Answer from the drawing. Dimensions are ordinates in mm from the lowest x, y and z of the part. A direction names the side the tool comes from. Coordinates: 2 decimals unless noted, no trailing zeros. Order: outer loops, then holes, each group sorted by start corner. A loop starts at its lowest first (then second) coordinate and runs counter-clockwise, first axis right, second up. Notation, with made-up numbers: M -34.5,6 L -30.5,6 A19 cw -30.5,34 Z; hole C -6,-26.75 d8. An arc over 180 degrees is marked long. One line per question, with ' | ' between items. Start each with the question number.
1) Find section A-A, the plane y = 5.61. Write down the section's boundary in (x, z).
2) Given P1, Ø7, axis at x = 19.31, y = 18.29, coming from the -Z side; P2, Ø3.5, axis at x = 6.63, y = 18.29, coming from the -Z side; P3, Ø6, axis at x = 25.5, z = 4, coming from the +Y side, each flat-ended and moving along its own axis, determine where each tip first touches the part or whether it passes through.
3) Find section B-B, the plane x = 31.99. Write down the section's boundary in (y, z), plus the area to 3 significant figures.
4) Consider probe 1 along Y at (x, z) = (31.99, 12.75); probe 2 along Z at (x, y) = (34, 21.75); probe 3 along Y at (x, z) = (25, 1.5). Determine where each line is inside the solid, lowest interval first.
5) Find section D-D, the plane x = 10. Write down the section's boundary in (y, z).
6) Find section C-C, the plane z = 8.25. Write down the section's boundary in (x, y).
7) A tool of negligible diameter and unlimited length cuts with its end or side. For the marked faces 1 and 2, from which of +Z, -Z, +X, -X, +Y, -Y can it reach the whole face along a straight path? Write none if from no direction.
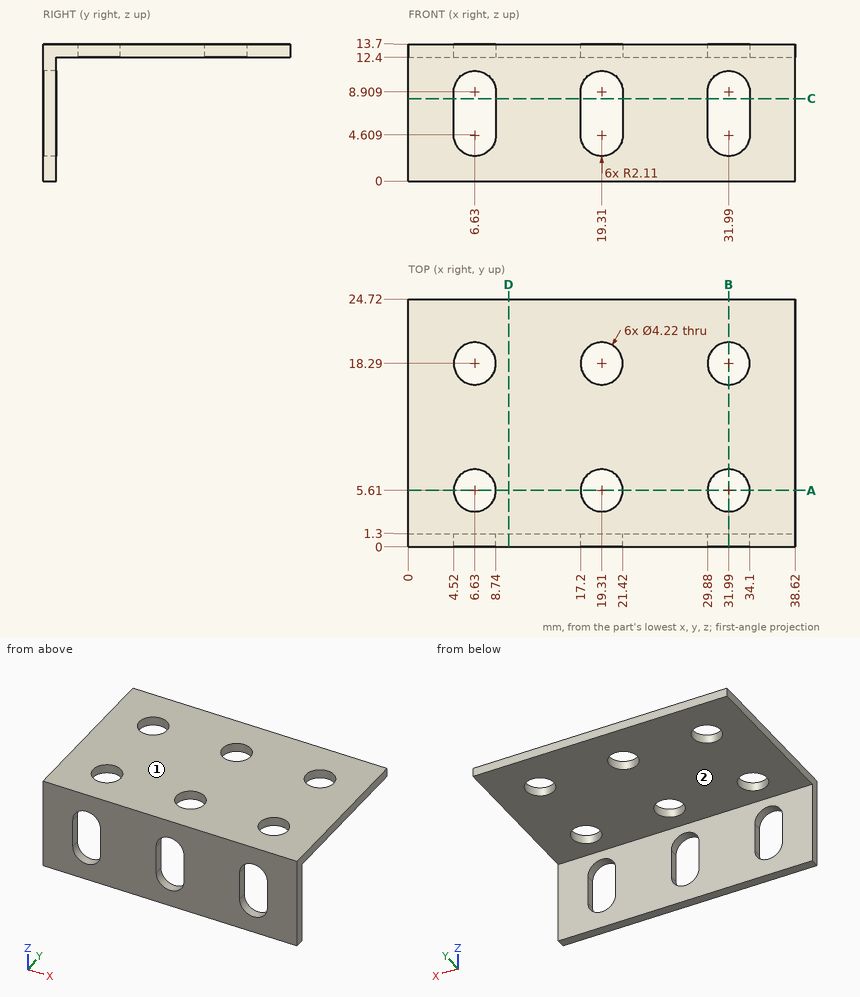
Report:
1) outline: M 0,12.4 L 4.52,12.4 L 4.52,13.7 L 0,13.7 Z; M 8.74,12.4 L 17.2,12.4 L 17.2,13.7 L 8.74,13.7 Z; M 21.42,12.4 L 29.88,12.4 L 29.88,13.7 L 21.42,13.7 Z; M 34.1,12.4 L 38.62,12.4 L 38.62,13.7 L 34.1,13.7 Z
2) P1: stops at z = 12.4 | P2: passes through | P3: stops at y = 1.3
3) outline: M 0,0 L 1.3,0 L 1.3,2.5 L 0,2.5 Z; M 0,11.02 L 1.3,11.02 L 1.3,12.4 L 3.5,12.4 L 3.5,13.7 L 0,13.7 Z; M 7.72,12.4 L 16.18,12.4 L 16.18,13.7 L 7.72,13.7 Z; M 20.4,12.4 L 24.72,12.4 L 24.72,13.7 L 20.4,13.7 Z | area: 26.2 mm^2
4) probe 1: y = 0 to 3.5, 7.72 to 16.18, 20.4 to 24.72 | probe 2: z = 12.4 to 13.7 | probe 3: y = 0 to 1.3
5) outline: M 0,0 L 1.3,0 L 1.3,12.4 L 24.72,12.4 L 24.72,13.7 L 0,13.7 Z
6) outline: M 0,0 L 4.52,0 L 4.52,1.3 L 0,1.3 Z; M 8.74,0 L 17.2,0 L 17.2,1.3 L 8.74,1.3 Z; M 21.42,0 L 29.88,0 L 29.88,1.3 L 21.42,1.3 Z; M 34.1,0 L 38.62,0 L 38.62,1.3 L 34.1,1.3 Z
7) face 1: +Z, +X, -X, +Y, -Y | face 2: -Z, +X, -X, +Y
